Autodesk Inventor part; units mm, degrees
ref_plane "Work Plane1" through (1.525, 0, 0) normal (0, 0, 1) x (1, 0, 0)
ref_plane "YZ Plane" through (0, 0, 0) normal (1, 0, 0) x (0, 1, 0)
ref_plane "XZ Plane" through (0, 0, 0) normal (0, 1, 0) x (-1, 0, 0)
sketch "Sketch1" plane through (0, 0, 0) normal (0, 0, 1) x (1, 0, 0)
  line L0 (0, 7.315) -> (0, 5)
  line L1 (4.5, 5) -> (20, 5)
  line L2 (20, 5) -> (20, 0)
  line L3 (20, 0) -> (-0.6001, 0)
  line L4 (-4.7201, 0) -> (24.12, 0)
  line L5 (-0.6001, 0) -> (-0.6001, 7.315)
  line L6 (-0.6001, 7.315) -> (0, 7.315)
  line L7 (4.5, 5) -> (3.5797, 5)
  line L8 (3.5797, 5) -> (0, 5)
  line L9 (0, -1.463) -> (0, 8.778)
  dimension "d0" = 20
  dimension "d1" = 15.5
  dimension "d2" = 10
  dimension "d9" = 0.6001
  dimension "d10" = 14.63
  dimension "d13" = 0.9203
  dimension "d14" = 10
revolve "Body" add sketch "Sketch1" angle 360 about axis through (20, 0, 0) along (-1, 0, 0)
sketch "Sketch2" plane through (-0.6001, 0, 0) normal (-1, 0, 0) x (0, 0, 1)
  line L0 (0, 9.2376) -> (8, 4.6188)
  line L1 (8, 4.6188) -> (8, -4.6188)
  line L2 (8, -4.6188) -> (0, -9.2376)
  line L3 (0, -9.2376) -> (-8, -4.6188)
  line L4 (-8, -4.6188) -> (-8, 4.6188)
  line L5 (-8, 4.6188) -> (0, 9.2376)
  point P0 (0, 0)
  point P1 (0, 0)
  dimension "d11" = 16
extrude "Head" add sketch "Sketch2" along normal blind 5.8
sketch "Sketch4" plane through (0, 0, 0) normal (0, 0, 1) x (1, 0, 0)
  line L0 (-6.4001, 8) -> (-6.4001, 9.2376)
  line L1 (-6.4001, 9.2376) -> (-5.6856, 9.2376)
  line L2 (-5.6856, 9.2376) -> (-6.4001, 8)
  line L3 (-7.5601, 0) -> (0.5599, 0)
  line L4 (-0.6001, 9.2376) -> (-6.4001, 9.2376)
  line L5 (-6.4001, 4.6188) -> (-6.4001, 9.2376)
  dimension "d5" = 30
  dimension "d19" = 16
revolve "Chamfer1" cut sketch "Sketch4" angle 360 about axis through (-10, 0, 0) along (1, 0, 0)
thread "Thread"
chamfer "Chamfer2" distance 0.9202 distance2 0.9203 1 edges at (20, -5, 0) measured on face at (20, -0.8193, 0.3214)
ref_plane "Work Plane1" through (1.525, 0, 0) normal (0, 0, 1) x (1, 0, 0)
equation "\"d0\" = NLG"
equation "\"d1\" = GEL"
equation "\"d2\" = GD"
equation "\"d10\" = SD2"
equation "\"d14\" = BDM"
equation "\"d11\" = SW"
equation "\"d3\" = KOH - SD"
equation "\"d5\" = ANG1"
equation "\"d19\" = SW0"
equation "\"d15\" = GEL"
equation "\"d6\" = -0.5 * SPD + 0.5 * GD"
equation "\"NLG\" = 20"
equation "\"GD\" = NND"
equation "\"BDM\" = NND"
equation "\"KOH\" = 6.4"
equation "\"GEL\" = 15.5"
equation "\"SW\" = 16"
equation "\"SW0\" = SW"
equation "\"SPD\" = NND - 1.2269 * PTC"
equation "\"SD2\" = 14.63"
equation "\"SD\" = 0.6"
equation "\"ANG1\" = 30deg"
equation "\"GAL\" = 0.61345 * PTC"
equation "\"GUL\" = 0.61345 * PTC"
equation "\"RR\" = 0.4"
equation "\"GD1\" = THREADDIA - 1.2269 * PTC"
equation "\"SDH\" = SD2"
equation "\"SDHG\" = 4.5"
equation "\"TOA\" = 30deg"
equation "\"PTC\" = 1.5"
equation "\"E0\" = 18.48"
properties part number "ISO 4017 - M10 x 20" material "Steel, Mild"
CAD build for the part. Positions are in the model's coordinates, mm. A direction names the side the tool comes from. Give positions to 0.01 mm unless a question says otherwise; leave off trailing zeros. Loops run counter-clockwise (first coordinate to the right, second up) from the corner with the lowest first, then second, coordinate; pieces in that order, holes last. Notation, with made-up numbers: (61, -28.75) -> (84, -28.75) arc R31 ccw to (84, -0.75) -> close; hole circle Ø5 at (20.25, 1.25). An arc over 180 degrees is marked (long way). Use a Markdown table: item, result.
1. Flat gauge pins, fed straight in: pin 1 (8 mm diameter, centred on x = 9, y = 0.5, fed in from -Z); pin 2 (1 mm diameter, centred on x = 4, z = -1, fed in from +Y); pin 3 (2 mm diameter, centred on x = 15, y = -5.5, fed in from -Z). Where does each tip first touch, or does it go through?
Check result:
| item | result |
|---|---|
| pin 1 | stops at z = -5 |
| pin 2 | stops at y = 4.97 |
| pin 3 | stops at z = -2.18 |
2. Wall check: L1, parallel to Y at x = -0.25, z = 0.25; L2, parallel to X at y = -0.5, z = 6; L3, parallel to X at y = -3, z = 7.25. Give the ranges that are in metal, low to high. Write a range as [from, to].
Check result:
| item | result |
|---|---|
| L1 | y = [-7.31, 7.31] |
| L2 | x = [-6.4, 0] |
| L3 | x = [-6.4, -0.6] |
3. Slice it at A-A (x = 10). List the corners of the cut face in (y, z).
Check result:
| item | result |
|---|---|
| outline | circle Ø10 at (0, 0) |
4. Which spindle directions (+Z, -Z, +X, -X, +Y, -Y) get a long thin tool onto all of the face, cutting with end or side? Do faces 1 (the flat face through (-0.6, -7, -3)), 2 (the flat face through (-3.46, -6.896, 4.056)). Say none if no direction does.
Check result:
| item | result |
|---|---|
| face 1 | +X |
| face 2 | +Z, +X, -X, -Y |
5. Slice it at B-B (x = -3.5). List the corners of the cut face in (y, z), plus the area to 3 significant figures.
Check result:
| item | result |
|---|---|
| outline | (-9.24, 0) -> (-4.62, -8) -> (4.62, -8) -> (9.24, 0) -> (4.62, 8) -> (-4.62, 8) -> close |
| area | 222 mm^2 |
